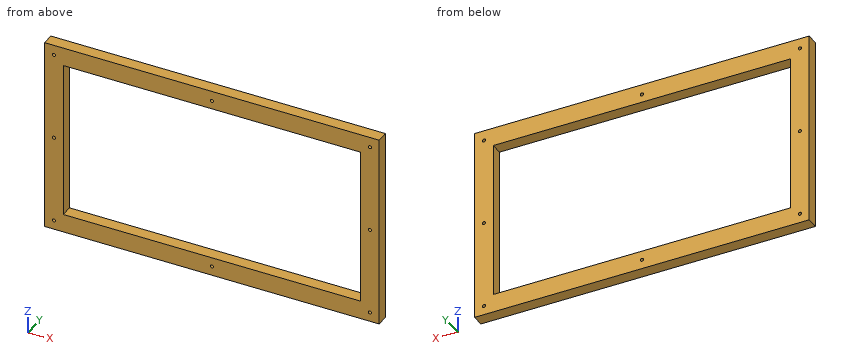
from build123d import *

# Parameters (mm, degrees)
SKETCH1_W                      = 358.27
SKETCH1_H                      = 211.05
BOSS_EXTRUDE1_DEPTH            = 12.7
SKETCH2_W                      = 318.27
SKETCH2_H                      = 171.05
CUT_EXTRUDE1_DEPTH             = 12.7
M3_CLEARANCE_HOLE1_D           = 3.4
M3_CLEARANCE_HOLE1_CSINK_D     = 3.45
M3_CLEARANCE_HOLE1_CSINK_ANGLE = 90


with BuildPart() as part:
    # Sketch1 → Boss-Extrude1 (new body)
    with BuildSketch(Plane(origin=(0, 0, 0), x_dir=(1, 0, 0), z_dir=(0, 1, 0))):
        Rectangle(SKETCH1_W, SKETCH1_H)
    extrude(amount=BOSS_EXTRUDE1_DEPTH)

    # Sketch2 → Cut-Extrude1 (cut)
    with BuildSketch(Plane(origin=(0, 12.7, 0), x_dir=(1, 0, 0), z_dir=(0, 1, 0))):
        Rectangle(SKETCH2_W, SKETCH2_H)
    extrude(amount=-CUT_EXTRUDE1_DEPTH, mode=Mode.SUBTRACT)

    # M3 Clearance Hole1 (through all)
    with Locations(Plane(origin=(0, 12.7, 0), x_dir=(1, 0, 0), z_dir=(0, 1, 0))):
        with Locations((-169.135, 95.525), (-169.135, 0.525), (-169.135, -94.475), (0, -94.475), (169.135, -94.475), (169.135, 0.525), (169.135, 95.525), (0, 95.525)):
            CounterSinkHole(M3_CLEARANCE_HOLE1_D / 2, M3_CLEARANCE_HOLE1_CSINK_D / 2, counter_sink_angle=M3_CLEARANCE_HOLE1_CSINK_ANGLE)


solid = part.part
Could you check a few things on this model? Use its own coordinates, in mm. Give positions to 0.01 mm unless a question says otherwise; leave off trailing zeros. Order: outer loops, then holes, each group sorted by start corner. A loop starts at its lowest first (then second) coordinate and runs counter-clockwise, first axis right, second up. Notation, with made-up numbers: (54, 2.5) -> (103, 2.5) arc R24 cw to (103, 28.5) -> close; hole circle Ø3 at (49.25, -3.75). An arc over 180 degrees is marked (long way). Return JSON: item names as keys, results as strings.
1. Imagine slicing it at A-A on x = 96. List the corners of the cut face in (y, z) for me (3 decimals), then the cut area to 3 significant figures.
Answer list:
{"outline": "(0, -105.525) -> (12.7, -105.525) -> (12.7, -85.525) -> (0, -85.525) -> close; (0, 85.525) -> (12.7, 85.525) -> (12.7, 105.525) -> (0, 105.525) -> close", "area": "508 mm2"}
2. Imagine slicing it at B-B on z = -57. List the corners of the cut face in (x, y) for me (3 decimals), then the cut area to 3 significant figures.
Answer list:
{"outline": "(-179.135, 0) -> (-159.135, 0) -> (-159.135, 12.7) -> (-179.135, 12.7) -> close; (159.135, 0) -> (179.135, 0) -> (179.135, 12.7) -> (159.135, 12.7) -> close", "area": "508 mm2"}
3. I need wall thicknesses on line 1 (Z direction, x = 0, y = 10) (3 decimals); line 2 (Z direction, x = -124, y = 6.5) (3 decimals); line 3 (X direction, y = 9.5, z = -48.5) (3 decimals). Which ranges of each line are inside material? Lowest first, please. Write a range as from..to.
Answer list:
{"line 1": "z = -105.525..-97.225, -93.825..-85.525, 85.525..92.775, 96.175..105.525", "line 2": "z = -105.525..-85.525, 85.525..105.525", "line 3": "x = -179.135..-159.135, 159.135..179.135"}
4. Imagine slicing it at C-C on y = 2.25. Give the number of separate pieces and of enclosed holes in the cut face, then the cut area to 3 significant figures.
Answer list:
{"separate pieces": "1", "enclosed holes": "9", "area": "21,100 mm2"}
5. For pin 1 Ø4 at (x, z) = (169.135, 94.475) entering from +Y; pin 2 Ø2 at (x, z) = (-169.135, -95.525) entering from -Y, each with a flat end and sliding along its axis, tell me the tip position at first contact or that it passes through.
Answer list:
{"pin 1": "stops at y = 12.7", "pin 2": "passes through"}
